Can you work these out from the model? Positions are in its coordinate system, mm. A direction names the side the tool comes from. Coordinates: 2 decimals unless noted, no trailing zeros. Order: outer loops, then holes, each group sorted by start corner. A loop starts at its lowest first (then second) coordinate and runs counter-clockwise, first axis right, second up. Notation, with made-up numbers: (51.5, 85.5) - (102.5, 85.5) arc R15 ccw to (102.5, 114.5) - close; hole circle Ø10 at (10, 19). An arc over 180 degrees is marked (long way). Return JSON: item names as keys, results as strings. Group by question number.
1) For pin 1 Ø2.5 at (x, z) = (-24, -2.5) entering from -Y; pin 2 Ø3.5 at (x, z) = (-1.5, 2) entering from +Y; pin 3 Ø4 at (y, z) = (-5.5, 0) entering from -X, each with a flat end and sliding along its axis, tell me the tip position at first contact or that it passes through.
2) Imagine slicing it at A-A (z = -3.25). Write out the boundary of the cut face in (x, y), and give its area (3 significant figures).
3) If I drill on line 1 along Z through (x, y) = (-15, -0.5); line 2 along Y through (x, z) = (-25.25, -2.35); line 3 along X through (y, z) = (-5.5, 0.95), over which ranges is the centre line in solid material (lowest first)?
4) Imagine slicing it at B-B (x = -21.5). Write out the boundary of the cut face in (y, z).
5) Imagine slicing it at C-C (x = -13). Write out the boundary of the cut face in (y, z).
6) If we mould it in two halves opening along Y, with no side actions, what happens to faces 1 (the face through (-4, -5, 0)), 2 (the face through (1, -6, 1.5)), 3 (the face through (-2, -3.5, 1))? For each: pulls with the +Y half, pulls with the -Y half, needs draft (parallel to the pull), parting line crosses it, or undercut.
7) Which directions (+Z, -Z, +X, -X, +Y, -Y) give clear straight access to the entire face, cutting with the end or side of a thin tool? Please do faces 4 (the face through (-0.197, -4.003, 2.26)), 5 (the face through (-24, 2.763, -3)), 6 (the face through (-0.17, -6.28, 0.74)).
```python
from build123d import *

# Parameters (mm, degrees)
BOSS_EXTRUDE1_DEPTH      = 3
BOSS_EXTRUDE1_DEPTH_BACK = 4.5
SKETCH1_R                = 0.8
FILLET1_R                = 4
CUT_EXTRUDE2_DEPTH       = 29.619267985
CUT_EXTRUDE2_DEPTH_BACK  = 29.619267985
SKETCH4_W                = 10.5
SKETCH4_H                = 4.5
CUT_EXTRUDE3_DEPTH       = 29.619267985
CUT_EXTRUDE3_DEPTH_BACK  = 29.619267985
SKETCH5_W                = 15
SKETCH5_H                = 4.5
FILLET2_R                = 10
FILLET3_R                = 5
FILLET4_R                = 5
CUT_EXTRUDE4_START       = -6.772335917
CUT_EXTRUDE4_DEPTH       = 8.772335917
SKETCH7_R                = 1.51
CUT_EXTRUDE5_DEPTH       = 1.5


# Read off the part's stored shape, not the designer's step: Cut-Extrude4
with BuildPart() as part:
    # Sketch1 → Boss-Extrude1 (new, two sides: drawn at the far end of the back side and taken through both)
    with BuildSketch(Plane.XY.offset(-BOSS_EXTRUDE1_DEPTH_BACK)):
        with BuildLine():
            Line((-4.389678411, -3.5), (-19.133343362, 6.422379894))
            ThreePointArc((-19.133343362, 6.422379894), (-19.666253628, 6.676053774), (-20.25, 6.763139721))
            Line((-20.25, 6.763139721), (-25.25, 6.763139721))
            ThreePointArc((-25.25, 6.763139721), (-27.246991207, 4.872803379), (-25.468997361, 2.775165839))
            ThreePointArc((-25.468997361, 2.775165839), (-25.359663658, 2.766148514), (-25.25, 2.763139721))
            Line((-25.25, 2.763139721), (-20.860321589, 2.763139721))
            Line((-20.860321589, 2.763139721), (-6.116656638, -7.159240173))
            ThreePointArc((-6.116656638, -7.159240173), (-5.583746372, -7.412914053), (-5, -7.5))
            Line((-5, -7.5), (0, -7.5))
            ThreePointArc((0, -7.5), (1.974370247, -5.81915847), (0.630136986, -3.601862129))
            ThreePointArc((0.630136986, -3.601862129), (0.31915847, -3.525629753), (0, -3.5))
            Line((0, -3.5), (-4.389678411, -3.5))
        make_face()
        with Locations((0, -5.5)):
            Circle(SKETCH1_R, mode=Mode.SUBTRACT)
        with Locations((-25.25, 4.763139721)):
            Circle(SKETCH1_R, mode=Mode.SUBTRACT)
    extrude(amount=BOSS_EXTRUDE1_DEPTH + BOSS_EXTRUDE1_DEPTH_BACK)

    # Fillet1
    fillet1_edges = [part.edges().sort_by_distance(p)[0] for p in [
        (-4.389678411, -3.5, -0.75),
        (-20.860321589, 2.763139721, -0.75),
    ]]
    fillet(fillet1_edges, radius=FILLET1_R)

    # Sketch4 → Cut-Extrude2 (cut, two sides: drawn at the far end of the back side and taken through both)
    with BuildSketch(Plane(origin=(0, 0, 0), x_dir=(1, 0, 0), z_dir=(0, 1, 0)).offset(-CUT_EXTRUDE2_DEPTH_BACK)):
        with Locations((-3.25, 2.25)):
            Rectangle(SKETCH4_W, SKETCH4_H)
    extrude(amount=CUT_EXTRUDE2_DEPTH + CUT_EXTRUDE2_DEPTH_BACK, mode=Mode.SUBTRACT)

    # Sketch5 → Cut-Extrude3 (cut, two sides: drawn at the far end of the back side and taken through both)
    with BuildSketch(Plane(origin=(0, 0, 0), x_dir=(1, 0, 0), z_dir=(0, 1, 0)).offset(-CUT_EXTRUDE3_DEPTH_BACK)):
        with Locations((-19.75, -0.75)):
            Rectangle(SKETCH5_W, SKETCH5_H)
    extrude(amount=CUT_EXTRUDE3_DEPTH + CUT_EXTRUDE3_DEPTH_BACK, mode=Mode.SUBTRACT)

    # Fillet2
    # the kernel refuses this fillet: 10 mm, written as the material it takes off along each edge
    with BuildSketch(Plane(origin=(-12.25, -23.910660804, 3), x_dir=(1.537930276954748e-12, 0, -1.0), z_dir=(0, 1, 0))) as fillet2_piece_1:
        with BuildLine():
            CenterArc((10, -8.351646544), FILLET2_R, 123.367012969, 56.632987031)
            Line((0, -8.351646544), (-0.2, -8.351646544))
            Line((-0.2, -8.351646544), (-0.2, 0))
            Line((-0.2, 0), (0, 0.2))
            ThreePointArc((0, 0.2), (2.25, 0.2), (4.39, 0.167032931))
            Line((4.39, 0.167032931), (4.5, 0))
        make_face()
    extrude(amount=46.579716753, mode=Mode.SUBTRACT)

    # Fillet3
    # the kernel refuses this fillet: 5 mm, written as the material it takes off along each edge
    with BuildSketch(Plane(origin=(-8.5, -17.99261029, -4.5), x_dir=(0, 0, 1), z_dir=(0, 1, 0))) as fillet3_piece_1:
        with BuildLine():
            CenterArc((5, -4.974937186), FILLET3_R, 95.739170477, 84.260829523)
            Line((0, -4.974937186), (-0.1, -4.974937186))
            Line((-0.1, -4.974937186), (-0.1, 0))
            Line((-0.1, 0), (0, 0.1))
            ThreePointArc((0, 0.1), (2.25, 0.1), (4.49, 0.099498744))
            Line((4.49, 0.099498744), (4.5, 0))
        make_face()
    extrude(amount=29.696169959, mode=Mode.SUBTRACT)

    # Fillet4
    fillet4_edges = [part.edges().sort_by_distance(p)[0] for p in [
        (-12.25, -0.620802428, -1.5),
    ]]
    fillet(fillet4_edges, radius=FILLET4_R)

    # Cut-Extrude4 outline → Cut-Extrude4 (cut)
    with BuildSketch(Plane(origin=(0, 0, 0), x_dir=(0, 0, -1), z_dir=(1, 0, 0)).offset(CUT_EXTRUDE4_START)):
        with BuildLine():
            add(Edge.make_bspline(
                [(-2.999498449, -5), (-2.961702123, -7.5), (-1.5, -7.5)],
                knots=[4.738249611, 4.738249611, 4.738249611, 6.283185307, 6.283185307, 6.283185307], degree=2, weights=[1, 0.716190529, 1]))
            Line((-2.999498449, -5), (-3, -5))
            Line((-3, -5), (-3, -7.5))
            Line((-3, -7.5), (-1.5, -7.5))
        make_face()
    extrude(amount=CUT_EXTRUDE4_DEPTH, mode=Mode.SUBTRACT)

    # Sketch7 → Cut-Extrude5 (cut)
    with BuildSketch(Plane.XY.offset(3)):
        with Locations((0, -5.5)):
            Circle(SKETCH7_R)
    extrude(amount=-CUT_EXTRUDE5_DEPTH, mode=Mode.SUBTRACT)


solid = part.part
```
Calculated:
{
 "1": {"pin 1": "y = 2.76", "pin 2": "y = -3.5", "pin 3": "x = -11.49"},
 "2": {"outline": "(-25.25, 2.76) - (-22.08, 2.76) arc R4 cw to (-19.85, 2.08) - (-10.17, -4.43) - (-10.17, 0.39) - (-19.13, 6.42) arc R2 ccw to (-20.25, 6.76) - (-25.25, 6.76) arc R2 ccw to start; hole circle Ø1.6 at (-25.25, 4.76)", "area": "73.0 mm2"},
 "3": {"line 1": "-4.5 to -1.5", "line 2": "2.76 to 3.96, 5.56 to 6.76", "line 3": "-8.58 to -0.8, 0.8 to 2"},
 "4": {"outline": "(2.72, -4.5) - (6.76, -4.5) - (6.76, -1.5) - (2.72, -1.5) - close"},
 "5": {"outline": "(-2.53, -4.48) - (2.29, -4.48) - (2.29, -1.23) - (-2.53, -1.23) - close"},
 "6": {"face 1": "needs draft", "face 2": "undercut", "face 3": "pulls with the +Y half"},
 "7": {"face 4": "+Z", "face 5": "+Z, -Z, -X, -Y", "face 6": "+Z, -Z"}
}
